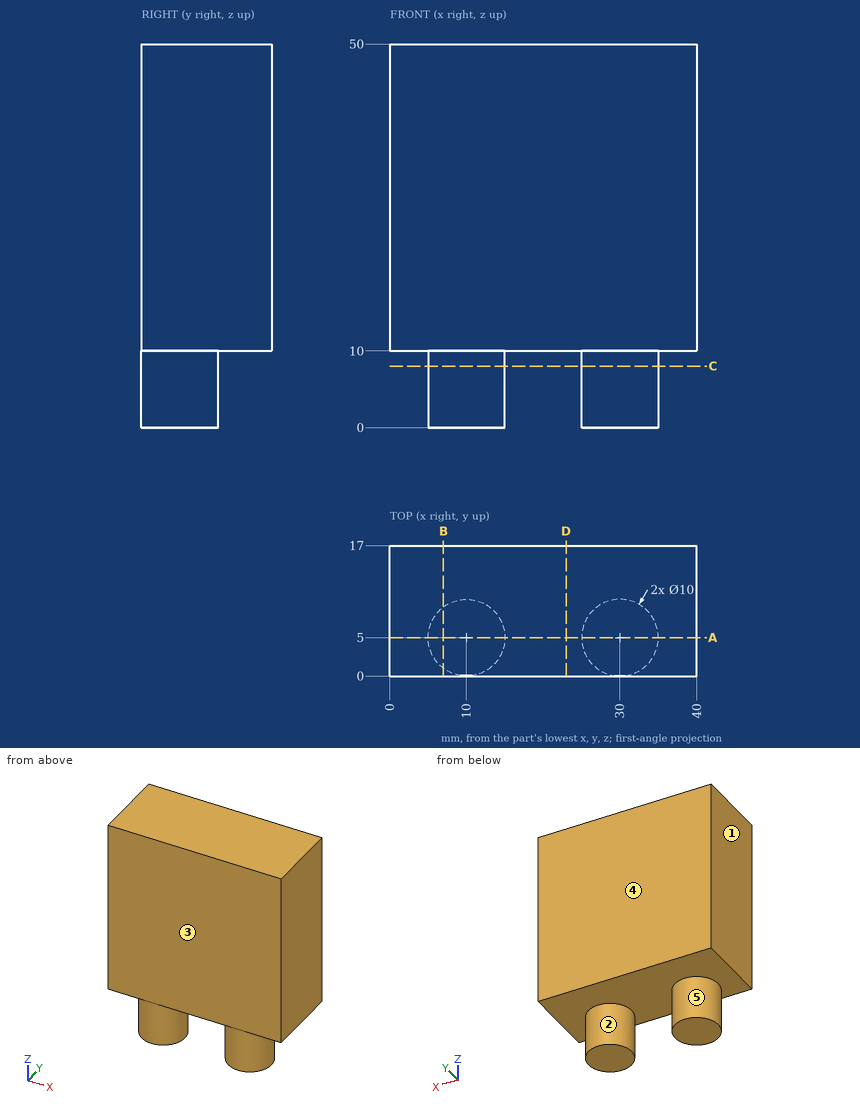
Input: dimensioned drawing with shaded views. Units: mm. Origin: part minimum x, y, z. A direction names the side the tool comes from. Coordinates: 2 decimals unless noted, no trailing zeros. Loops run counter-clockwise (first coordinate to the right, second up) from the corner with the lowest first, then second, coordinate; pieces in that order, holes last.
Q1. Mould query, pull axis X, two halves, no side actions, for the marked faces 1, 2 and 3. Classes: +X half, -X half, draft (parallel to the pull), parting line (faces both ways), or undercut.
Results are:
face 1: -X half
face 2: undercut
face 3: draft
Q2. Section A-A, the plane y = 5. Return the cut outline in (x, z).
Results are:
outline: (0, 10) - (5, 10) - (5, 0) - (15, 0) - (15, 10) - (25, 10) - (25, 0) - (35, 0) - (35, 10) - (40, 10) - (40, 50) - (0, 50) - close
Q3. Section B-B, the plane x = 7. Return the cut outline in (y, z), and give its area (3 significant figures).
Results are:
outline: (0, 10) - (1, 10) - (1, 0) - (9, 0) - (9, 10) - (17, 10) - (17, 50) - (0, 50) - close
area: 760 mm2
Q4. Set-up query: the marked faces 4 and 5. Return all of +Z, -Z, +X, -X, +Y, -Y with unobstructed straight access to the full face (end or side cutting, diameter ignored); none if empty.
Results are:
face 4: +Z, -Z, +X, -X, +Y
face 5: -Z
Q5. Section C-C, the plane z = 8. Return the cut outline in (x, y), and give its area (3 significant figures).
Results are:
outline: circle Ø10 at (10, 5); circle Ø10 at (30, 5)
area: 157 mm2
Q6. Section D-D, the plane x = 23. Return the cut outline in (y, z).
Results are:
outline: (0, 10) - (17, 10) - (17, 50) - (0, 50) - close
Q7. Line query: line 1 along Z through (x, y) = (37, 1.25); line 2 along X through (y, z) = (9.25, 9). Output: solid intervals per line, ascending.
Results are:
line 1: z = 10 to 50
line 2: x = 7.37 to 12.63, 27.37 to 32.63
